Can you work these out from the drawing? Everything is in mm from the part's minimum corner. Give positions to 0.01 mm unless a question says otherwise; leave off trailing zeros. Order: outer loops, then holes, each group sorted by start corner. A loop starts at its lowest first (then second) coordinate and runs counter-clockwise, first axis right, second up. Notation, with made-up numbers: M -27.75,-4 L 9.25,-4 A16 ccw 9.25,14 Z; hole C 3,7.25 d11. An arc over 180 degrees is marked long. Use a Markdown table: item, result. Add a question column.
Item 1: Suppose I cut it at A-A on y = 55. Write out the boundary of the cut face in (x, z).
Item 2: Suppose I cut it at D-D on y = 84. Write out the boundary of the cut face in (x, z).
Item 3: If I drill on L1, parallel to Y at x = 25, z = 3.7; L2, parallel to X at y = 55, z = 2.85; L3, parallel to Y at x = 18, z = 2.3, over which ranges is the centre line in solid material (lowest first)? Write a range as from..to.
Item 4: I'm going to push flat-ended pins straight in: pin 1 Ø17.5 at (x, y) = (25, 55) entering from +Z; pin 2 Ø1.5 at (x, z) = (56.5, 2.5) entering from -Y. Where does each tip first touch, or does it pass through?
Item 5: Suppose I cut it at C-C on z = 3.7. Write out the boundary of the cut face in (x, y).
Item 6: Suppose I cut it at B-B on x = 25. Write out the boundary of the cut face in (y, z).
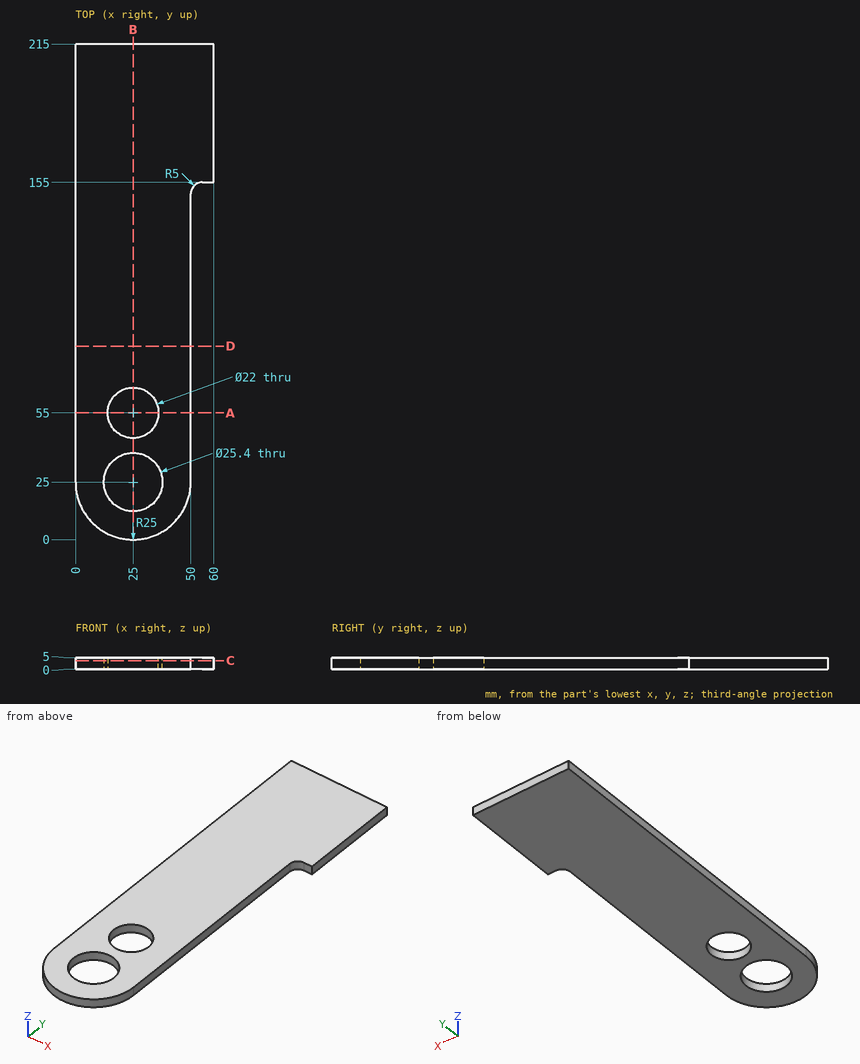
Findings below:
| question | item | result |
|---|---|---|
| 1 | outline | M 0,0 L 14,0 L 14,5 L 0,5 Z; M 36,0 L 50,0 L 50,5 L 36,5 Z |
| 2 | outline | M 0,0 L 50,0 L 50,5 L 0,5 Z |
| 3 | L1 | y = 0..12.3, 37.7..44, 66..215 |
| 3 | L2 | x = 0..14, 36..50 |
| 3 | L3 | y = 1..14.4, 35.6..46.51, 63.49..215 |
| 4 | pin 1 | passes through |
| 4 | pin 2 | stops at y = 155 |
| 5 | outline | M 0,25 A25 ccw 50,25 L 50,150 A5 cw 55,155 L 60,155 L 60,215 L 0,215 Z; hole C 25,25 d25.4; hole C 25,55 d22 |
| 6 | outline | M 0,0 L 12.3,0 L 12.3,5 L 0,5 Z; M 37.7,0 L 44,0 L 44,5 L 37.7,5 Z; M 66,0 L 215,0 L 215,5 L 66,5 Z |
